Input: dimensioned drawing with shaded views. Units: mm. Origin: part minimum x, y, z. Round coordinates to 2 decimals unless told otherwise and drop trailing zeros. Order: outer loops, then holes, each group sorted by start corner. A loop starts at its lowest first (then second) coordinate and runs counter-clockwise, first axis right, second up. Notation, with made-up numbers: (-6.75, 17) - (44.25, 17) arc R25 ccw to (44.25, 40) - close; hole circle Ø8 at (27, 73.25). An arc over 180 degrees is marked (long way). Return JSON: item names as keys, results as strings. Group by question number.
1) Section D-D, the plane x = 15. Return loops of the section in (y, z), plus the area to 3 significant figures.
2) Section A-A, the plane y = 17.5. Return loops of the section in (x, z) (1 decimal).
3) Section C-C, the plane z = 0.55. Give the number of separate pieces and of enclosed holes in the cut face, plus the area to 3 significant figures.
4) Contact query for flat-ended pins moving along their axis: P1, Ø8, axis at x = 9.5, y = 21.5, coming from the -Z side; P2, Ø5.5, axis at x = 65, y = 17.5, coming from the -Z side. Output: stop coordinate, or through.
5) Section B-B, the plane x = 40. Return loops of the section in (y, z) (3 decimals).
6) Ray query, line 1 (Y direction, x = 15, z = 0.8); line 2 (Y direction, x = 65, z = 1.2); line 3 (X direction, y = 19.5, z = 1.65). Return the intervals inside material, ascending. Write a range as from..to.
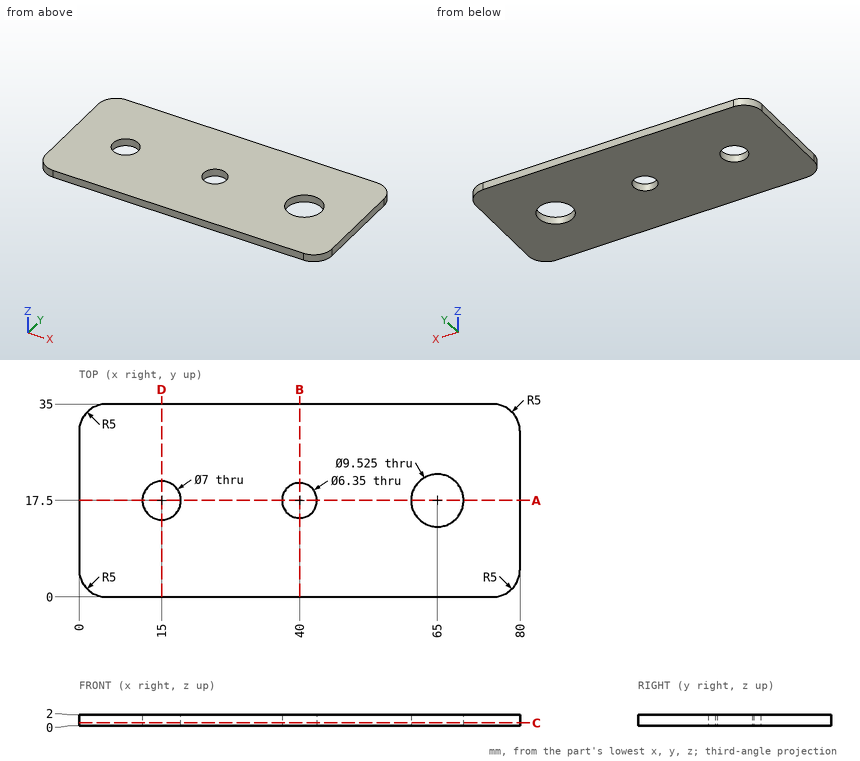
Geometry check:
{
 "1": {"outline": "(0, 0) - (14, 0) - (14, 2) - (0, 2) - close; (21, 0) - (35, 0) - (35, 2) - (21, 2) - close", "area": "56.0 mm2"},
 "2": {"outline": "(0, 0) - (11.5, 0) - (11.5, 2) - (0, 2) - close; (18.5, 0) - (36.8, 0) - (36.8, 2) - (18.5, 2) - close; (43.2, 0) - (60.2, 0) - (60.2, 2) - (43.2, 2) - close; (69.8, 0) - (80, 0) - (80, 2) - (69.8, 2) - close"},
 "3": {"separate pieces": "1", "enclosed holes": "3", "area": "2,640 mm2"},
 "4": {"P1": "z = 0", "P2": "through"},
 "5": {"outline": "(0, 0) - (14.325, 0) - (14.325, 2) - (0, 2) - close; (20.675, 0) - (35, 0) - (35, 2) - (20.675, 2) - close"},
 "6": {"line 1": "0..14, 21..35", "line 2": "0..12.74, 22.26..35", "line 3": "0..12.13, 17.87..37.53, 42.47..60.68, 69.32..80"}
}
